Check sheet for the modelled part. Datum: model origin and axes. Units: mm. A direction names the side the tool comes from. Give positions to 0.01 mm unless a question says otherwise; leave off trailing zeros. Write each loop counter-clockwise with the first axis right and the second up, starting at its lowest first coordinate (ties: lowest second). Pieces come first, ordered by that corner, then holes.
from build123d import *

# Parameters (mm, degrees)
SKETCH2_R           = 4.5
BOSS_EXTRUDE1_DEPTH = 5
SKETCH3_W           = 5
SKETCH3_H           = 0.741657387
BOSS_EXTRUDE2_DEPTH = 8
CUT_EXTRUDE1_REACH  = 18.037
SKETCH4_R           = 1
SKETCH6_R           = 2
CUT_EXTRUDE2_DEPTH  = 5


with BuildPart() as part:
    # Sketch2 → Boss-Extrude1 (new body)
    with BuildSketch(Plane(origin=(0, 0, 0), x_dir=(1, 0, 0), z_dir=(0, 1, 0))):
        with Locations(Location((0, 0, 0), (0, 0, 270))):
            Circle(SKETCH2_R)
    extrude(amount=BOSS_EXTRUDE1_DEPTH)

    # Sketch3 → Boss-Extrude2 (add)
    with BuildSketch(Plane(origin=(0, 5, 0), x_dir=(1, 0, 0), z_dir=(0, 1, 0))):
        with Locations((0, -3.370828694)):
            Rectangle(SKETCH3_W, SKETCH3_H)
        with Locations((0, 3.370828694)):
            Rectangle(SKETCH3_W, SKETCH3_H)
    extrude(amount=BOSS_EXTRUDE2_DEPTH)

    # Cut-Extrude1: up to this face of the body (flat: up to its plane)
    cut_extrude1_end = Plane(part.part.faces().sort_by_distance((0, 9, -3.741657387))[0])
    # Sketch4 → Cut-Extrude1 (cut, up to the picked face)
    with BuildSketch(Plane.XY.offset(3.741657387), mode=Mode.PRIVATE) as cut_extrude1_sk1:
        with Locations((0, 11.5)):
            Circle(SKETCH4_R)
    cut_extrude1_tool1 = split(extrude(cut_extrude1_sk1.sketch, amount=-CUT_EXTRUDE1_REACH, mode=Mode.PRIVATE), bisect_by=cut_extrude1_end, keep=Keep.BOTH, mode=Mode.PRIVATE)
    add(cut_extrude1_tool1.solids().sort_by(Axis((0, 11.5, 3.741657), (0, 0, -1)))[0], mode=Mode.SUBTRACT)

    # Sketch6 → Cut-Extrude2 (cut)
    with BuildSketch(Plane.XZ):
        with Locations(Location((0, 0, 0), (0, 0, 270))):
            Circle(SKETCH6_R)
    extrude(amount=-CUT_EXTRUDE2_DEPTH, mode=Mode.SUBTRACT)

    # Sketch9 → M3x0.5 Tapped Hole2 (revolve, cut)
    with BuildSketch(Plane(origin=(0, 2.5, 4.5), x_dir=(0, -1, 0), z_dir=(1, 0, 0))):
        Polygon((0, 0), (0, 4.499), (1.25, 3.747924226), (1.25, 0), align=None)
    m3x0_5_tapped_hole2 = revolve(axis=Axis((0, 2.5, 10.85), (0, 0, -1)), mode=Mode.SUBTRACT)

    # Mirror1: M3x0.5 Tapped Hole2 across plane
    add(m3x0_5_tapped_hole2.mirror(Plane.XY), mode=Mode.SUBTRACT)


solid = part.part
1) Draft check along Z on faces 1 (the flat face through (0, 9, 3.742)), 2 (the cylindrical face through (2, 2, 0)), 3 (the cylindrical face through (0.46, 10.61, -3.37)), 4 (the cylindrical face through (-1.72, 2.46, 4.16)). Enter one of: +Z half, -Z half, draft (parallel to the pull), parting line (faces both ways), or undercut.
2) Sectioned sample at D-D on z = -2.75. Record the boundary of the cut face in (x, y).
3) Gauge pin test, flat ends, axial feed: pin 1 (0.6 mm diameter, centred on y = 7, z = 3, fed in from -X); pin 2 (4 mm diameter, centred on x = 3.5, y = 9, fed in from +Z); pin 3 (0.8 mm diameter, centred on x = 0.5, z = 4, fed in from +Y); pin 4 (2.5 mm diameter, centred on x = -0.5, y = 11, fed in from -Z). Record the tip position at first contact, or that the pin passes through.
4) Access from +Z, -Z, +X, -X, +Y, -Y to the whole of each face (thin tool, end or side, straight path). Record for faces 5 (the cylindrical face through (0.46, 10.61, 3.38)), 6 (the flat face through (0, 9, 3)), 7 (the flat face through (0, 9, -3.742)).
5) Scan lines: L1, parallel to Y at x = 0, z = 3.2; L2, parallel to Z at x = 2, y = 6.75; L3, parallel to X at y = 2.3, z = 0. Record each from-to range of solid material in increasing order.
6) Sectioned sample at B-B on y = 7.75. Record the boundary of the cut face in (x, z), then the cut area to 3 significant figures.
7) Sectioned sample at C-C on y = 11.5. Record the boundary of the cut face in (x, z).
8) Sectioned sample at A-A on z = 0. Record the boundary of the cut face in (x, y), then the cut area to 3 significant figures.
Answers below:
1. face 1: +Z half
1. face 2: undercut
1. face 3: draft
1. face 4: parting line
2. outline: (-3.56, 0) - (3.56, 0) - (3.56, 5) - (-3.56, 5) - close; hole circle Ø2.5 at (0, 2.5)
3. pin 1: stops at x = -2.5
3. pin 2: stops at z = 3.74
3. pin 3: stops at y = 13
3. pin 4: stops at z = -3.74
4. face 5: +Z, -Z
4. face 6: +X, -X, +Y
4. face 7: -Z, +X, -X, +Y
5. L1: y = 0 to 1.25, 3.75 to 10.5, 12.5 to 13
5. L2: z = -3.74 to -3, 3 to 3.74
5. L3: x = -4.5 to -2, 2 to 4.5
6. outline: (-2.5, -3.74) - (2.5, -3.74) - (2.5, -3) - (-2.5, -3) - close; (-2.5, 3) - (2.5, 3) - (2.5, 3.74) - (-2.5, 3.74) - close
6. area: 7.42 mm2
7. outline: (-2.5, -3.74) - (-1, -3.74) - (-1, -3) - (-2.5, -3) - close; (-2.5, 3) - (-1, 3) - (-1, 3.74) - (-2.5, 3.74) - close; (1, -3.74) - (2.5, -3.74) - (2.5, -3) - (1, -3) - close; (1, 3) - (2.5, 3) - (2.5, 3.74) - (1, 3.74) - close
8. outline: (-4.5, 0) - (-2, 0) - (-2, 5) - (-4.5, 5) - close; (2, 0) - (4.5, 0) - (4.5, 5) - (2, 5) - close
8. area: 25.0 mm2
